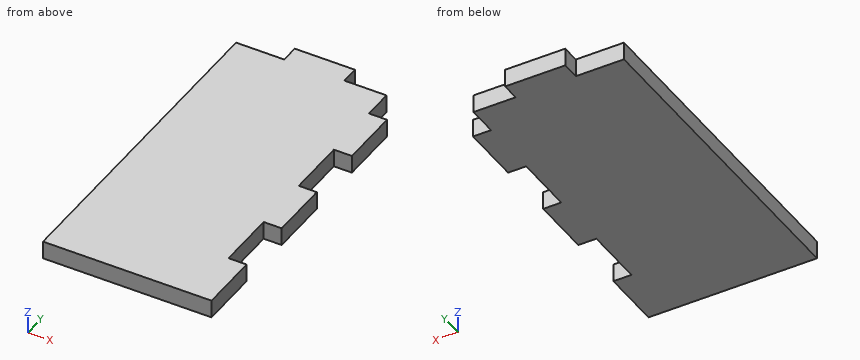
```python
from build123d import *

# Parameters (mm, degrees)
ESQUISSE1_W                = 28
ESQUISSE1_H                = 58
BOSS_EXTRU_1_DEPTH         = 3
ESQUISSE2_W                = 10
ESQUISSE2_H                = 3
ENL_V_MAT_EXTRU_1_DEPTH    = 3
R_P_TITION_LIN_AIRE1_COUNT = 2
R_P_TITION_LIN_AIRE1_PITCH = 20
ESQUISSE3_W                = 3
ESQUISSE3_H                = 10
ENL_V_MAT_EXTRU_2_DEPTH    = 3
R_P_TITION_LIN_AIRE2_COUNT = 3
R_P_TITION_LIN_AIRE2_PITCH = 20


with BuildPart() as part:
    # Esquisse1 → Boss.-Extru.1 (new body)
    with BuildSketch(Plane.XY):
        with Locations((14, -29)):
            Rectangle(ESQUISSE1_W, ESQUISSE1_H)
    extrude(amount=BOSS_EXTRU_1_DEPTH)

    # Esquisse2 → Enlèv. mat.-Extru.1 (cut)
    with BuildSketch(Plane.XY.offset(3)):
        with Locations((23, -1.5)):
            Rectangle(ESQUISSE2_W, ESQUISSE2_H)
    enl_v_mat_extru_1 = extrude(amount=-ENL_V_MAT_EXTRU_1_DEPTH, mode=Mode.SUBTRACT)

    # Répétition linéaire1: Enlèv. mat.-Extru.1 ×2
    with Locations(*[(-i * R_P_TITION_LIN_AIRE1_PITCH, 0, 0) for i in range(1, R_P_TITION_LIN_AIRE1_COUNT)]):
        add(enl_v_mat_extru_1, mode=Mode.SUBTRACT)

    # Esquisse3 → Enlèv. mat.-Extru.2 (cut)
    with BuildSketch(Plane.XY.offset(3)):
        with Locations((26.5, -43)):
            Rectangle(ESQUISSE3_W, ESQUISSE3_H)
    enl_v_mat_extru_2 = extrude(amount=-ENL_V_MAT_EXTRU_2_DEPTH, mode=Mode.SUBTRACT)

    # Répétition linéaire2: Enlèv. mat.-Extru.2 ×3
    with Locations(*[(0, i * R_P_TITION_LIN_AIRE2_PITCH, 0) for i in range(1, R_P_TITION_LIN_AIRE2_COUNT)]):
        add(enl_v_mat_extru_2, mode=Mode.SUBTRACT)


solid = part.part
```
Geometry: final body of the model. Coordinates: model frame, mm. Coordinates: 2 decimals unless noted, no trailing zeros. Order: outer loops, then holes, each group sorted by start corner. A loop starts at its lowest first (then second) coordinate and runs counter-clockwise, first axis right, second up. Notation, with made-up numbers: (85.25, 28.5) -> (128.25, 28.5) arc R15 ccw to (128.25, 38.5) -> close; hole circle Ø6 at (-4.5, 38). An arc over 180 degrees is marked (long way). Write item = value, one per line.
(1) Cut plane A-A on x = 26. Return loops of the section in (y, z), plus the area to 3 significant figures.
Solved:
outline = (-58, 0) -> (-48, 0) -> (-48, 3) -> (-58, 3) -> close; (-38, 0) -> (-28, 0) -> (-28, 3) -> (-38, 3) -> close; (-18, 0) -> (-8, 0) -> (-8, 3) -> (-18, 3) -> close
area = 90.0 mm²
(2) Cut plane B-B on z = 1.75. Return loops of the section in (x, y), plus the area to 4 significant figures.
Solved:
outline = (0, -58) -> (28, -58) -> (28, -48) -> (25, -48) -> (25, -38) -> (28, -38) -> (28, -28) -> (25, -28) -> (25, -18) -> (28, -18) -> (28, -8) -> (25, -8) -> (25, -3) -> (18, -3) -> (18, 0) -> (8, 0) -> (8, -3) -> (0, -3) -> close
area = 1,495 mm²
(3) Cut plane C-C on y = -44. Return loops of the section in (x, z).
Solved:
outline = (0, 0) -> (25, 0) -> (25, 3) -> (0, 3) -> close
(4) Line query: line 1 (Y direction, x = 19.5, z = 2.2); line 2 (X direction, y = -40, z = 0.6); line 3 (X direction, y = -2.5, z = 0.2). Output: solid intervals per line, ascending.
Solved:
line_1 = -58 to -3
line_2 = 0 to 25
line_3 = 8 to 18
(5) Pin query (flat end, axial travel): pin 1 Ø8 at (x, y) = (17.5, -31.5) entering from -Z; pin 2 Ø0.9 at (y, z) = (-23.5, 1.5) entering from +X; pin 3 Ø1.5 at (x, z) = (23, 2) entering from +Y; pin 4 Ø1.5 at (x, z) = (27, 1) entering from +Y. Return the tip coordinate at first contact, or that it passes through.
Solved:
pin_1 = 0
pin_2 = 25
pin_3 = -3
pin_4 = -8
(6) Cut plane D-D on x = 19.5. Return loops of the section in (y, z), plus the area to 3 significant figures.
Solved:
outline = (-58, 0) -> (-3, 0) -> (-3, 3) -> (-58, 3) -> close
area = 165 mm²
